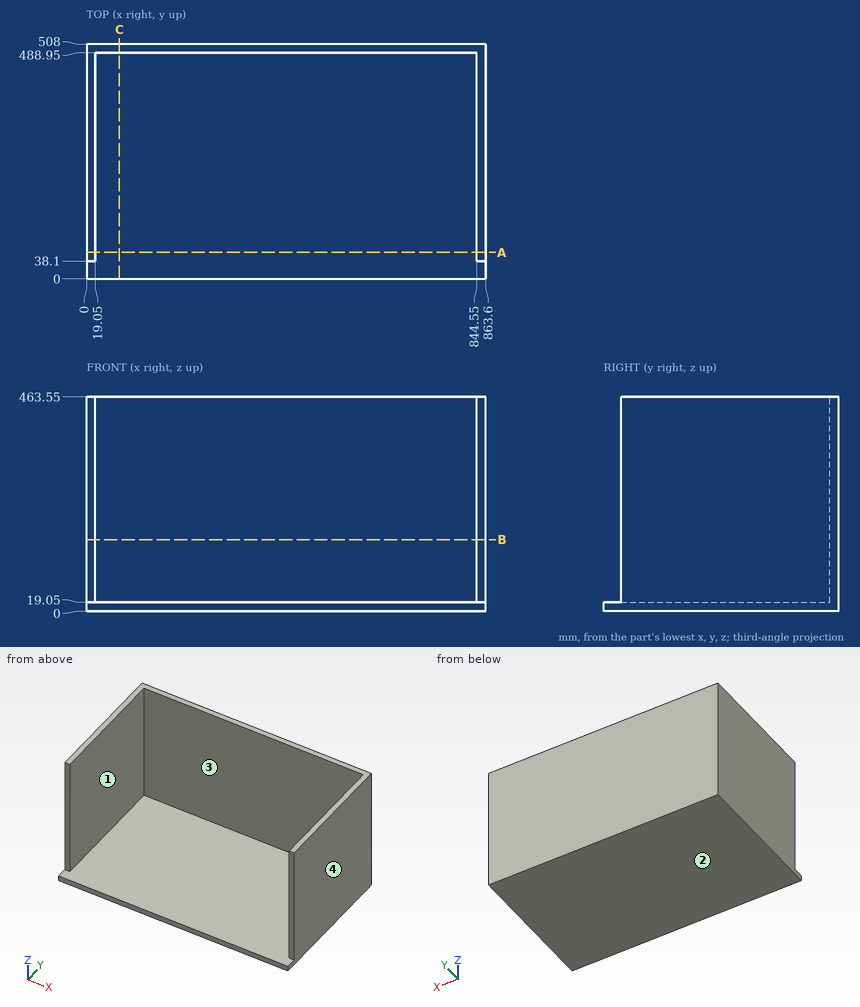
The figure shows three views and two pictorial views of one solid part (mm, origin at its lowest corner). Answer the questions. Round coordinates to 2 decimals unless told otherwise and drop trailing zeros. Write each loop counter-clockwise with the first axis right and the second up, starting at its lowest first coordinate (ties: lowest second). Pieces come first, ordered by that corner, then holes. Notation, with made-up numbers: (5.25, 25) -> (30.25, 25) arc R29 ccw to (30.25, 47) -> close; hole circle Ø10 at (-22.5, 40.5). An arc over 180 degrees is marked (long way). Answer as a JSON object with one key per item and string values. Group by question number.
Q1. Section B-B (z = 154.5) is taken. Write down the section's boundary in (x, y).
Q2. Straight lines are drawn through the part: line 1 along X through (y, z) = (231, 273); line 2 along Y through (x, z) = (504.5, 182); line 3 along Z through (x, y) = (166.5, 476). For each, find the intervals that lie inside material, in ascending order.
Q3. Section A-A (y = 57) is taken. Write down the section's boundary in (x, z).
Q4. Determine the mould class of the marked faces 1, 2, 3 and 4 for opening direction X: pulls with the +X half, pulls with the -X half, needs draft (parallel to the pull), parting line crosses it, or undercut.
Q5. Each of these flat-tipped pins is pushed along its axis until it touches: pin 1 Ø8 at (x, y) = (564.5, 288) entering from -Z; pin 2 Ø4 at (x, y) = (638, 198) entering from +Z; pin 3 Ø9.5 at (x, z) = (851.5, 204.5) entering from -Y. Where does it stop, or does it pass through?
Q6. Section C-C (x = 71) is taken. Write down the section's boundary in (y, z).
Check values:
{
 "1": {"outline": "(0, 38.1) -> (19.05, 38.1) -> (19.05, 488.95) -> (844.55, 488.95) -> (844.55, 38.1) -> (863.6, 38.1) -> (863.6, 508) -> (0, 508) -> close"},
 "2": {"line 1": "0 to 19.05, 844.55 to 863.6", "line 2": "488.95 to 508", "line 3": "0 to 19.05"},
 "3": {"outline": "(0, 0) -> (863.6, 0) -> (863.6, 463.55) -> (844.55, 463.55) -> (844.55, 19.05) -> (19.05, 19.05) -> (19.05, 463.55) -> (0, 463.55) -> close"},
 "4": {"face 1": "undercut", "face 2": "needs draft", "face 3": "undercut", "face 4": "pulls with the +X half"},
 "5": {"pin 1": "z = 0", "pin 2": "z = 19.05", "pin 3": "y = 38.1"},
 "6": {"outline": "(0, 0) -> (508, 0) -> (508, 463.55) -> (488.95, 463.55) -> (488.95, 19.05) -> (0, 19.05) -> close"}
}
